Can you work these out from the model? Positions are in its coordinate system, mm. Coordinates: 2 decimals unless noted, no trailing zeros. Loops run counter-clockwise (first coordinate to the right, second up) from the corner with the lowest first, then second, coordinate; pieces in that order, holes last. Notation, with made-up numbers: (35, -33.75) -> (43, -33.75) arc R26 ccw to (43, -15.75) -> close; hole circle Ø4 at (3, 47.5). An arc over 180 degrees is marked (long way). Use one line per item in the form item = value. Start each with the question number.
(1) Imagine slicing it at A-A (z = -21.25). List the corners of the cut face in (x, y) for me.
(2) Imagine slicing it at C-C (x = 21.75). List the corners of the cut face in (y, z) for me.
(3) I need wall thicknesses on line 1 (X direction, y = 1.5, z = -16); line 2 (X direction, y = 0.9, z = -21.25); line 3 (X direction, y = 0.15, z = 9). Which ranges of each line are inside material? Lowest first, please. Write a range as [from, to].
(4) I'm going to push a flat-ended pin straight in: pin 1 (0.8 mm diameter, centred on y = 0.5, z = -7.5, fed in from -X). Where does the tip first touch, or does it pass through?
(5) Imagine slicing it at D-D (z = -12.5). List the corners of the cut face in (x, y) for me.
(6) Imagine slicing it at B-B (x = -10). List the corners of the cut face in (y, z) for me, plus the area to 3 significant figures.
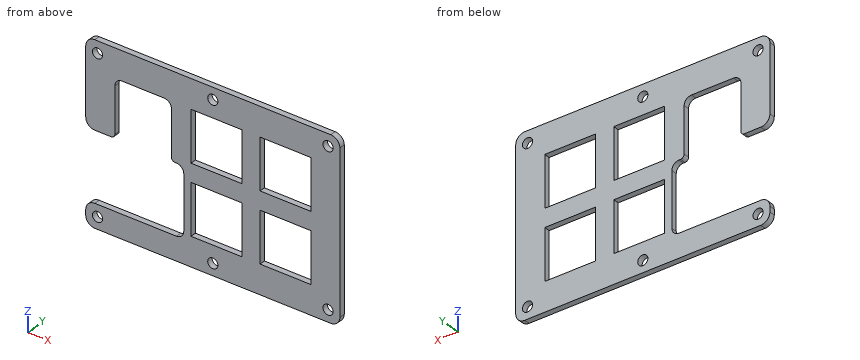
```python
from build123d import *

# Parameters (mm, degrees)
SKETCH1_W            = 40
SKETCH1_H            = 39
BOSS_EXTRUDE1_DEPTH  = 1.6
SKETCH3_W            = 70
SKETCH3_H            = 49
BOSS_EXTRUDE2_DEPTH  = 1.6
SKETCH4_W            = 27
SKETCH4_H            = 19
CUT_EXTRUDE1_DEPTH   = 2.6
FILLET1_R            = 2
SKETCH5_W            = 15.6
SKETCH5_H            = 15.6
CUT_EXTRUDE2_DEPTH   = 2.6
FILLET2_R            = 2
FILLET3_R            = 1
SKETCH6_R            = 1.4
CUT_EXTRUDE3_DEPTH   = 2.6
FILLET4_R            = 2.5
SKETCH7_W            = 14
SKETCH7_H            = 14
CUT_EXTRUDE4_DEPTH   = 2.6
LPATTERN1_COUNT      = 2
LPATTERN1_PITCH      = 19
LPATTERN1_COUNT_DIR2 = 2
LPATTERN1_PITCH_DIR2 = 19


with BuildPart() as part:
    # Sketch1 → Boss-Extrude1 (new body)
    with BuildSketch(Plane(origin=(0, 0, 0), x_dir=(1, 0, 0), z_dir=(0, 1, 0))):
        Rectangle(SKETCH1_W, SKETCH1_H)
    extrude(amount=BOSS_EXTRUDE1_DEPTH)

    # Sketch3 → Boss-Extrude2 (add)
    with BuildSketch(Plane(origin=(0, 0, 0), x_dir=(1, 0, 0), z_dir=(0, 1, 0))):
        with Locations((-10, 0)):
            Rectangle(SKETCH3_W, SKETCH3_H)
    extrude(amount=BOSS_EXTRUDE2_DEPTH)

    # Sketch4 → Cut-Extrude1 (cut, through all)
    with BuildSketch(Plane(origin=(0, 1.6, 0), x_dir=(1, 0, 0), z_dir=(0, 1, 0))):
        with Locations((-31.5, 8.5)):
            Rectangle(SKETCH4_W, SKETCH4_H)
    extrude(amount=-CUT_EXTRUDE1_DEPTH, mode=Mode.SUBTRACT)

    # Fillet1
    fillet1_edges = [part.edges().sort_by_distance(p)[0] for p in [
        (-18, 0.8, -18),
        (-18, 0.8, 1),
    ]]
    fillet(fillet1_edges, radius=FILLET1_R)

    # Sketch5 → Cut-Extrude2 (cut, through all)
    with BuildSketch(Plane(origin=(0, 1.6, 0), x_dir=(1, 0, 0), z_dir=(0, 1, 0))):
        with Locations((-29.2, -8.8)):
            Rectangle(SKETCH5_W, SKETCH5_H)
    extrude(amount=-CUT_EXTRUDE2_DEPTH, mode=Mode.SUBTRACT)

    # Fillet2
    fillet2_edges = [part.edges().sort_by_distance(p)[0] for p in [
        (-37, 0.8, 16.6),
        (-21.4, 0.8, 16.6),
    ]]
    fillet(fillet2_edges, radius=FILLET2_R)

    # Fillet3
    fillet3_edges = [part.edges().sort_by_distance(p)[0] for p in [
        (-37, 0.8, 1),
        (-21.4, 0.8, 1),
    ]]
    fillet(fillet3_edges, radius=FILLET3_R)

    # Sketch6 → Cut-Extrude3 (cut, through all)
    with BuildSketch(Plane(origin=(0, 1.6, 0), x_dir=(1, 0, 0), z_dir=(0, 1, 0))):
        with Locations((-41.75, 21.25)):
            Circle(SKETCH6_R)
        with Locations((21.75, 21.25)):
            Circle(SKETCH6_R)
        with Locations((21.75, -21.25)):
            Circle(SKETCH6_R)
        with Locations((-41.75, -21.25)):
            Circle(SKETCH6_R)
        with Locations((-10, -21.25)):
            Circle(SKETCH6_R)
        with Locations((-10, 21.25)):
            Circle(SKETCH6_R)
    extrude(amount=-CUT_EXTRUDE3_DEPTH, mode=Mode.SUBTRACT)

    # Fillet4
    fillet4_edges = [part.edges().sort_by_distance(p)[0] for p in [
        (25, 0.8, 24.5),
        (25, 0.8, -24.5),
        (-45, 0.8, -24.5),
        (-45, 0.8, 24.5),
        (-45, 0.8, 1),
        (-45, 0.8, -18),
    ]]
    fillet(fillet4_edges, radius=FILLET4_R)

    # Sketch7 → Cut-Extrude4 (cut, through all)
    with BuildSketch(Plane(origin=(0, 1.6, 0), x_dir=(1, 0, 0), z_dir=(0, 1, 0))):
        with Locations((-9, 9.5)):
            Rectangle(SKETCH7_W, SKETCH7_H)
    cut_extrude4 = extrude(amount=-CUT_EXTRUDE4_DEPTH, mode=Mode.SUBTRACT)

    # LPattern1: Cut-Extrude4 2 × 2
    with Locations(*[(i * LPATTERN1_PITCH, 0, j * LPATTERN1_PITCH_DIR2) for i in range(LPATTERN1_COUNT) for j in range(LPATTERN1_COUNT_DIR2) if (i, j) != (0, 0)]):
        add(cut_extrude4, mode=Mode.SUBTRACT)


solid = part.part
```
Worked out:
q1.outline = (-45, 0) -> (-43.15, 0) -> (-43.15, 1.6) -> (-45, 1.6) -> close; (-40.35, 0) -> (-11.4, 0) -> (-11.4, 1.6) -> (-40.35, 1.6) -> close; (-8.6, 0) -> (20.35, 0) -> (20.35, 1.6) -> (-8.6, 1.6) -> close; (23.15, 0) -> (25, 0) -> (25, 1.6) -> (23.15, 1.6) -> close
q2.outline = (0, -24.5) -> (1.6, -24.5) -> (1.6, -22.65) -> (0, -22.65) -> close; (0, -19.85) -> (1.6, -19.85) -> (1.6, 19.85) -> (0, 19.85) -> close; (0, 22.65) -> (1.6, 22.65) -> (1.6, 24.5) -> (0, 24.5) -> close
q3.line_1 = [-18, -16], [-2, 3], [17, 25]
q3.line_2 = [-45, -43.15], [-40.35, -11.4], [-8.6, 20.35], [23.15, 25]
q3.line_3 = [-45, -37], [-21.4, -16], [-2, 3], [17, 25]
q4.pin_1 = -18
q5.outline = (-18, 0) -> (-16, 0) -> (-16, 1.6) -> (-18, 1.6) -> close; (-2, 0) -> (3, 0) -> (3, 1.6) -> (-2, 1.6) -> close; (17, 0) -> (25, 0) -> (25, 1.6) -> (17, 1.6) -> close
q6.outline = (0, -24.5) -> (1.6, -24.5) -> (1.6, -22.65) -> (0, -22.65) -> close; (0, -19.85) -> (1.6, -19.85) -> (1.6, -16.5) -> (0, -16.5) -> close; (0, -2.5) -> (1.6, -2.5) -> (1.6, 2.5) -> (0, 2.5) -> close; (0, 16.5) -> (1.6, 16.5) -> (1.6, 19.85) -> (0, 19.85) -> close; (0, 22.65) -> (1.6, 22.65) -> (1.6, 24.5) -> (0, 24.5) -> close
q6.area = 24.6 mm2
